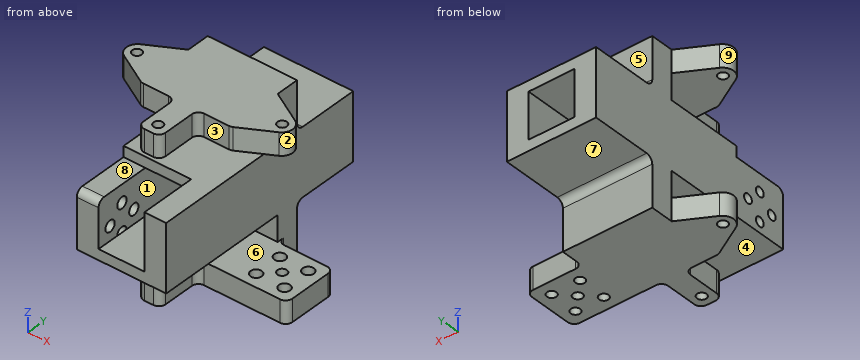
from build123d import *

# Parameters (mm, degrees)
SKETCH2_W           = 40
SKETCH2_H           = 30
BOSS_EXTRUDE1_DEPTH = 100
SKETCH3_W           = 20.5
SKETCH3_H           = 20.5
CUT_EXTRUDE1_DEPTH  = 100
SKETCH4_W           = 20.5
SKETCH4_H           = 50
CUT_EXTRUDE2_DEPTH  = 4.75
SKETCH5_W           = 4.75
SKETCH5_H           = 25
CUT_EXTRUDE4_DEPTH  = 9.75
SKETCH6_R           = 2.1
CUT_EXTRUDE5_DEPTH  = 9.75
SKETCH7_R           = 2.5
CUT_EXTRUDE6_DEPTH  = 5.18
SKETCH8_W           = 40
SKETCH8_H           = 10.38
BOSS_EXTRUDE2_DEPTH = 21.5
SKETCH9_W           = 40
SKETCH9_H           = 10
BOSS_EXTRUDE3_DEPTH = 45
BOSS_EXTRUDE4_START = -65
SKETCH11_W          = 10
SKETCH11_H          = 25
BOSS_EXTRUDE4_DEPTH = 90
SKETCH13_R          = 2.1
CUT_EXTRUDE7_DEPTH  = 4.57
SKETCH14_R          = 2.1
SKETCH14_R_2        = 2.5
CUT_EXTRUDE8_DEPTH  = 5.43
SKETCH15_R          = 2.1
CUT_EXTRUDE9_DEPTH  = 10
CUT_EXTRUDE10_REACH = 133.735
SKETCH18_R          = 2.1
SKETCH19_W          = 15
SKETCH19_H          = 20.005
CUT_EXTRUDE11_DEPTH = 12.57
FILLET1_R           = 3


with BuildPart() as part:
    # Sketch2 → Boss-Extrude1 (new body)
    with BuildSketch(Plane(origin=(0, 0, 0), x_dir=(1, 0, 0), z_dir=(0, 1, 0))):
        Rectangle(SKETCH2_W, SKETCH2_H)
    extrude(amount=BOSS_EXTRUDE1_DEPTH)

    # Sketch3 → Cut-Extrude1 (cut)
    with BuildSketch(Plane(origin=(0, 0, 0), x_dir=(1, 0, 0), z_dir=(0, 1, 0))):
        Rectangle(SKETCH3_W, SKETCH3_H)
    extrude(amount=CUT_EXTRUDE1_DEPTH, mode=Mode.SUBTRACT)

    # Sketch4 → Cut-Extrude2 (cut)
    with BuildSketch(Plane.XY.offset(15)):
        Rectangle(SKETCH4_W, SKETCH4_H)
    extrude(amount=-CUT_EXTRUDE2_DEPTH, mode=Mode.SUBTRACT)

    # Sketch5 → Cut-Extrude4 (cut)
    with BuildSketch(Plane(origin=(-10.25, 0, 0), x_dir=(0, 0, -1), z_dir=(1, 0, 0))):
        with Locations((-12.625, 12.5)):
            Rectangle(SKETCH5_W, SKETCH5_H)
    extrude(amount=-CUT_EXTRUDE4_DEPTH, mode=Mode.SUBTRACT)

    # Sketch6 → Cut-Extrude5 (cut)
    with BuildSketch(Plane.ZY.offset(20)):
        with Locations((2.425, 12.5)):
            Circle(SKETCH6_R)
        with Locations((-10.275, 12.5)):
            Circle(SKETCH6_R)
        with Locations((-3.925, 18.85)):
            Circle(SKETCH6_R)
        with Locations((-3.925, 6.15)):
            Circle(SKETCH6_R)
    extrude(amount=-CUT_EXTRUDE5_DEPTH, mode=Mode.SUBTRACT)

    # Sketch7 → Cut-Extrude6 (cut)
    with BuildSketch(Plane(origin=(-10.25, 0, 0), x_dir=(0, 0, -1), z_dir=(1, 0, 0))):
        with Locations((-2.425, 12.5)):
            Circle(SKETCH7_R)
        with Locations((10.275, 12.5)):
            Circle(SKETCH7_R)
        with Locations((3.925, 18.85)):
            Circle(SKETCH7_R)
        with Locations((3.925, 6.15)):
            Circle(SKETCH7_R)
    extrude(amount=-CUT_EXTRUDE6_DEPTH, mode=Mode.SUBTRACT)

    # Sketch8 → Boss-Extrude2 (add)
    with BuildSketch(Plane(origin=(0, 0, -15), x_dir=(-1, 0, 0), z_dir=(0, 0, -1))):
        with Locations((0, 64.81)):
            Rectangle(SKETCH8_W, SKETCH8_H)
    boss_extrude2 = extrude(amount=BOSS_EXTRUDE2_DEPTH)

    # Sketch9 → Boss-Extrude3 (add)
    with BuildSketch(Plane.XZ.offset(-59.62)):
        with Locations((0, -31.5)):
            Rectangle(SKETCH9_W, SKETCH9_H)
    boss_extrude3 = extrude(amount=BOSS_EXTRUDE3_DEPTH)

    # Sketch11 → Boss-Extrude4 (add)
    with BuildSketch(Plane(origin=(20, 0, 0), x_dir=(0, 0, -1), z_dir=(1, 0, 0)).offset(BOSS_EXTRUDE4_START)):
        with Locations((31.5, 47.125)):
            Rectangle(SKETCH11_W, SKETCH11_H)
    boss_extrude4 = extrude(amount=BOSS_EXTRUDE4_DEPTH)

    # Sketch13 → Cut-Extrude7 (cut)
    with BuildSketch(Plane(origin=(0, 0, -36.5), x_dir=(-1, 0, 0), z_dir=(0, 0, -1))):
        with Locations((-32.5, 47.125)):
            Circle(SKETCH13_R)
        with Locations((-26.15, 53.475)):
            Circle(SKETCH13_R)
        with Locations((-38.85, 53.475)):
            Circle(SKETCH13_R)
        with Locations((-38.85, 40.775)):
            Circle(SKETCH13_R)
        with Locations((-26.15, 40.775)):
            Circle(SKETCH13_R)
    extrude(amount=-CUT_EXTRUDE7_DEPTH, mode=Mode.SUBTRACT)

    # Sketch14 → Cut-Extrude8 (cut)
    with BuildSketch(Plane.XY.offset(-26.5)):
        with Locations(Location((32.5, 47.125, 0), (0, 0, 180))):
            Circle(SKETCH14_R)
        with Locations((38.85, 53.475)):
            Circle(SKETCH14_R_2)
        with Locations((26.15, 53.475)):
            Circle(SKETCH14_R_2)
        with Locations((26.15, 40.775)):
            Circle(SKETCH14_R_2)
        with Locations((38.85, 40.775)):
            Circle(SKETCH14_R_2)
    extrude(amount=-CUT_EXTRUDE8_DEPTH, mode=Mode.SUBTRACT)

    # Sketch15 → Cut-Extrude9 (cut)
    with BuildSketch(Plane(origin=(0, 0, -36.5), x_dir=(-1, 0, 0), z_dir=(0, 0, -1))):
        with Locations((32.5, 47.125)):
            Circle(SKETCH15_R)
        with Locations((0, 19.65)):
            Circle(SKETCH15_R)
        with BuildLine():
            Line((20, 59.625), (34.632584515, 51.495786381))
            ThreePointArc((34.632584515, 51.495786381), (37.204369859, 47.125), (34.632584515, 42.754213619))
            Line((34.632584515, 42.754213619), (20, 34.625))
            Line((20, 34.625), (45, 34.625))
            Line((45, 34.625), (45, 59.625))
            Line((45, 59.625), (20, 59.625))
        make_face()
    cut_extrude9 = extrude(amount=-CUT_EXTRUDE9_DEPTH, mode=Mode.SUBTRACT)

    # Mirror2: Boss-Extrude2, Boss-Extrude3, Boss-Extrude4, Cut-Extrude9 across plane
    add(boss_extrude2.mirror(Plane.XY))
    add(boss_extrude3.mirror(Plane.XY))
    add(boss_extrude4.mirror(Plane.XY))
    add(cut_extrude9.mirror(Plane.XY), mode=Mode.SUBTRACT)

    # Sketch18 → Cut-Extrude10 (cut, up to next)
    with BuildSketch(Plane.XY.offset(36.5), mode=Mode.PRIVATE) as cut_extrude10_sk1:
        with BuildLine():
            Line((20, 59.625), (34.632584515, 51.495786381))
            ThreePointArc((34.632584515, 51.495786381), (37.204369859, 47.125), (34.632584515, 42.754213619))
            Line((34.632584515, 42.754213619), (20, 34.625))
            Line((20, 34.625), (45, 34.625))
            Line((45, 34.625), (45, 59.625))
            Line((45, 59.625), (20, 59.625))
        make_face()
    cut_extrude10_tool1 = extrude(cut_extrude10_sk1.sketch, amount=-CUT_EXTRUDE10_REACH, mode=Mode.PRIVATE) & part.part
    # Sketch18 → Cut-Extrude10 (cut, up to next)
    with BuildSketch(Plane.XY.offset(36.5), mode=Mode.PRIVATE) as cut_extrude10_sk2:
        with Locations(Location((32.5, 47.125, 0), (0, 0, 180))):
            Circle(SKETCH18_R)
    cut_extrude10_tool2 = extrude(cut_extrude10_sk2.sketch, amount=-CUT_EXTRUDE10_REACH, mode=Mode.PRIVATE) & part.part
    add(cut_extrude10_tool1.solids().sort_by_distance((27.487993, 55.869454, 36.5))[0], mode=Mode.SUBTRACT)
    add(cut_extrude10_tool2.solids().sort_by_distance((32.5, 47.125, 36.5))[0], mode=Mode.SUBTRACT)

    # Sketch19 → Cut-Extrude11 (cut)
    with BuildSketch(Plane.XY.offset(36.5)):
        with Locations((-12.5, 24.6225)):
            Rectangle(SKETCH19_W, SKETCH19_H)
        with Locations((12.5, 24.6225)):
            Rectangle(SKETCH19_W, SKETCH19_H)
    cut_extrude11 = extrude(amount=-CUT_EXTRUDE11_DEPTH, mode=Mode.SUBTRACT)

    # Mirror3: Cut-Extrude11 across plane
    add(cut_extrude11.mirror(Plane.XY), mode=Mode.SUBTRACT)

    # Fillet1
    fillet1_edges = [part.edges().sort_by_distance(p)[0] for p in [
        (0, 70, -15),
        (20, 59.625, -31.5),
        (-20, 34.625, -31.5),
        (45, 34.625, -31.5),
        (45, 59.625, -31.5),
        (0, 70, 15),
        (20, 34.625, 31.5),
        (-20, 34.625, 31.5),
        (5, 14.62, 31.5),
        (-5, 14.62, 31.5),
        (-5, 34.625, 31.5),
        (5, 34.625, 31.5),
        (5, 14.62, -31.5),
        (-5, 14.62, -31.5),
        (-5, 34.625, -31.5),
        (5, 34.625, -31.5),
        (-15.125, 0, 10.25),
    ]]
    fillet(fillet1_edges, radius=FILLET1_R)


solid = part.part
Verification items for the finished model (mm, model axes). Face numbers are marked on the shaded views. A direction names the side the tool comes from. Coordinates: 2 decimals unless noted, no trailing zeros. Order: outer loops, then holes, each group sorted by start corner. A loop starts at its lowest first (then second) coordinate and runs counter-clockwise, first axis right, second up. Notation, with made-up numbers: M -19.5,70 L 0.5,70 A23 cw 0.5,104 Z; hole C -15.75,13 d6. An arc over 180 degrees is marked long. Return JSON: item names as keys, results as strings.
1) Cross-section at A-A, the plane y = 6.15. Record the boundary of the cut face in (x, z) (3 decimals), and give its area (3 significant figures).
Answer list:
{"outline": "M -20,-15 L 20,-15 L 20,15 L 10.25,15 L 10.25,-10.25 L -10.25,-10.25 L -10.25,-6.425 L -15.43,-6.425 L -15.43,-6.025 L -20,-6.025 Z; M -20,-1.825 L -15.43,-1.825 L -15.43,-1.425 L -10.25,-1.425 L -10.25,10.25 L -20,10.25 Z", "area": "591 mm2"}
2) Cross-section at B-B, the plane y = 79.5. Record the boundary of the cut face in (x, z), and give its area (3 significant figures).
Answer list:
{"outline": "M -20,-15 L 20,-15 L 20,15 L -20,15 Z; hole M -10.25,-10.25 L 10.25,-10.25 L 10.25,10.25 L -10.25,10.25 Z", "area": "780 mm2"}
3) Gauge pin test, flat ends, axial feed: pin 1 (4 mm diameter, centred on y = 12.5, z = 2.425, fed in from -X); pin 2 (8 mm diameter, centred on y = 29.5, z = -4.5, fed in from -X); pin 3 (5 mm diameter, centred on x = -13, z = 32.5, fed in from -Y) (3 decimals). Record the tip position at first contact, or that the pin passes through.
Answer list:
{"pin 1": "x = 10.25", "pin 2": "x = -20", "pin 3": "y = 34.625"}
4) Thickness scan on L1, parallel to Y at x = 26, z = -33 (3 decimals); L2, parallel to Y at x = 26.15, z = -29 (3 decimals); L3, parallel to Z at x = -17, y = 12. Record the ranges inside material, lowest first. Write a range as [from, to].
Answer list:
{"L1": "[34.625, 38.68], [42.87, 51.38], [55.57, 59.625]", "L2": "[34.625, 38.275], [43.275, 50.975], [55.975, 59.625]", "L3": "[-15, -12.31], [-8.24, 0.39], [4.46, 10.25]"}
5) Cross-section at D-D, the plane x = 32. Record the boundary of the cut face in (y, z) (3 decimals), and give its area (3 significant figures).
Answer list:
{"outline": "M 34.625,-36.5 L 45.085,-36.5 L 45.085,-26.5 L 34.625,-26.5 Z; M 41.292,26.5 L 45.085,26.5 L 45.085,36.5 L 41.292,36.5 Z; M 49.165,-36.5 L 59.625,-36.5 L 59.625,-26.5 L 49.165,-26.5 Z; M 49.165,26.5 L 52.958,26.5 L 52.958,36.5 L 49.165,36.5 Z", "area": "285 mm2"}
6) Access from +Z, -Z, +X, -X, +Y, -Y to the whole of each face (thin tool, end or side, straight path). Record for the marked faces 1, 2, 3, 4 and 5.
Answer list:
{"face 1": "+Y, -Y", "face 2": "+Z, +X", "face 3": "+Z, +X, -Y", "face 4": "+X, -X, -Y", "face 5": "+Z, +X, -X, +Y"}
7) Cross-section at C-C, the plane x = 0. Count the separate pieces of the cut face and the enclosed holes in it, and give its area (3 significant figures).
Answer list:
{"separate pieces": "4", "enclosed holes": "0", "area": "2,100 mm2"}
8) Release check for a two-part mould opening along Z. For the marked faces 6, 7, 8 and 9 record: +Z half, -Z half, draft (parallel to the pull), parting line (faces both ways), or undercut.
Answer list:
{"face 6": "undercut", "face 7": "-Z half", "face 8": "+Z half", "face 9": "draft"}
